Here's how the part is built. I have some questions about the finished solid (model axes, mm). Face numbers are marked on the shaded views. A direction names the side the tool comes from. Coordinates: 2 decimals unless noted, no trailing zeros. Write each loop counter-clockwise with the first axis right and the second up, starting at its lowest first coordinate (ties: lowest second). Pieces come first, ordered by that corner, then holes.
Item 1: If we section it at D-D (z = -2.75): Please give me the cut outline in (x, y).
Item 2: If I drill on line 1 (Y direction, x = 0.5, z = -3); line 2 (Y direction, x = -1.5, z = 4.5); line 3 (X direction, y = 4.25, z = -1.5), over which ranges is the centre line in solid material (lowest first)?
Item 3: I'm going to push flat-ended pins straight in: pin 1 Ø6 at (x, z) = (3.5, -2.5) entering from +Y; pin 2 Ø1 at (x, y) = (-0.5, 5) entering from -Z; pin 3 Ø1 at (x, y) = (0.5, 6) entering from +Z; pin 4 Ø1.6 at (y, z) = (5.5, -1) entering from +X. Where does each tip first touch, or does it pass through?
Item 4: For the marked faces 1, 2, 3, 4 and 5, which set-ups out of +Z, -Z, +X, -X, +Y, -Y let a thin tool reach every point of the face, with its end or its side?
Item 5: If we section it at B-B (x = 0): Please give me the cut outline in (y, z), then the cut area to 3 significant figures.
Item 6: If we section it at A-A (z = 0): Please give me the cut outline in (x, y), then the cut area to 3 significant figures.
Item 7: If we section it at C-C (y = 6): Please give me the cut outline in (x, z), then the cut area to 3 significant figures.
from build123d import *

# Parameters (mm, degrees)
SKETCH1_W           = 12
SKETCH1_H           = 12
BOSS_EXTRUDE1_DEPTH = 3
SKETCH3_R           = 3.5
BOSS_EXTRUDE2_DEPTH = 1
SKETCH4_W           = 3.8
SKETCH4_H           = 3.8
BOSS_EXTRUDE3_DEPTH = 3.2


with BuildPart() as part:
    # Sketch1 → Boss-Extrude1 (new body)
    with BuildSketch(Plane(origin=(0, 0, 0), x_dir=(1, 0, 0), z_dir=(0, 1, 0))):
        Rectangle(SKETCH1_W, SKETCH1_H)
    extrude(amount=BOSS_EXTRUDE1_DEPTH)

    # Sketch3 → Boss-Extrude2 (add)
    with BuildSketch(Plane(origin=(0, 3, 0), x_dir=(1, 0, 0), z_dir=(0, 1, 0))):
        Circle(SKETCH3_R)
    extrude(amount=BOSS_EXTRUDE2_DEPTH)

    # Sketch4 → Boss-Extrude3 (add)
    with BuildSketch(Plane(origin=(0, 4, 0), x_dir=(1, 0, 0), z_dir=(0, 1, 0))):
        Rectangle(SKETCH4_W, SKETCH4_H)
    extrude(amount=BOSS_EXTRUDE3_DEPTH)


solid = part.part
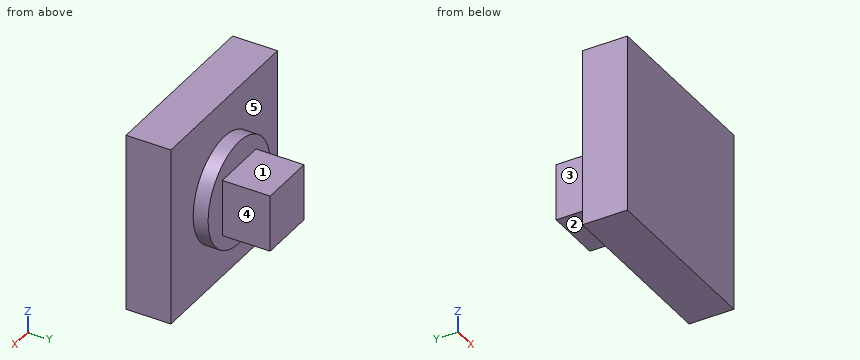
Answer list:
1. outline: (-6, 0) - (6, 0) - (6, 3) - (2.17, 3) - (2.17, 4) - (-2.17, 4) - (-2.17, 3) - (-6, 3) - close
2. line 1: y = 0 to 4
2. line 2: y = 0 to 3
2. line 3: x = -1.9 to 1.9
3. pin 1: stops at y = 7.2
3. pin 2: stops at z = -1.9
3. pin 3: stops at z = 1.9
3. pin 4: stops at x = 1.9
4. face 1: +Z, +X, -X, +Y
4. face 2: -Z, +X, -X, +Y
4. face 3: +Z, -Z, -X, +Y
4. face 4: +Z, -Z, +X, +Y
4. face 5: +Y
5. outline: (0, -6) - (3, -6) - (3, -3.5) - (4, -3.5) - (4, -1.9) - (7.2, -1.9) - (7.2, 1.9) - (4, 1.9) - (4, 3.5) - (3, 3.5) - (3, 6) - (0, 6) - close
5. area: 55.2 mm2
6. outline: (-6, 0) - (6, 0) - (6, 3) - (3.5, 3) - (3.5, 4) - (1.9, 4) - (1.9, 7.2) - (-1.9, 7.2) - (-1.9, 4) - (-3.5, 4) - (-3.5, 3) - (-6, 3) - close
6. area: 55.2 mm2
7. outline: (-1.9, -1.9) - (1.9, -1.9) - (1.9, 1.9) - (-1.9, 1.9) - close
7. area: 14.4 mm2
